Autodesk Inventor part; units mm, degrees
ref_plane "YZ Plane" through (0, 0, 0) normal (1, 0, 0) x (0, 1, 0)
ref_plane "XZ Plane" through (0, 0, 0) normal (0, 1, 0) x (-1, 0, 0)
ref_plane "XY Plane" through (0, 0, 0) normal (0, 0, 1) x (1, 0, 0)
sketch "Sketch1" plane through (0, 0, 0) normal (1, 0, 0) x (0, 1, 0)
  line L0 (0, 0) -> (15, 0)
  line L1 (15, 0) -> (12.3428, -7.0424)
  line L2 (12.3428, -7.0424) -> (2.9628, -13.5)
  line L3 (2.9628, -13.5) -> (-16.504, -16)
  line L4 (-16.504, -16) -> (-16.504, -11)
  line L5 (-16.504, -11) -> (-7.6685, -9.267)
  line L6 (-7.6685, -9.267) -> (-2.3251, -6.639)
  line L7 (-2.3251, -6.639) -> (0, 0)
  dimension "d0" = 15
  dimension "d24" = 16
  dimension "d27" = 5
extrude "Extrusion1" add sketch "Sketch1" along normal blind 20
sketch "Sketch2" plane through (0, 0, 0) normal (0, 0, 1) x (1, 0, 0)
  line L0 (-0.936, -0.2322) -> (7.6821, -18.3326)
  line L1 (7.6821, -18.3326) -> (-7.1135, -18.3326)
  line L2 (-7.1135, -18.3326) -> (-0.936, -0.2322)
extrude "Extrusion2" cut sketch "Sketch2" against normal blind 25
shell "Shell1" thickness 0.8 removed faces 2 at (6.6667, 5, 0) at (11.2076, -16.504, -14.3333)
sketch "Sketch3" plane through (0, 0, 0) normal (0, 0, 1) x (1, 0, 0)
  line L0 (0.8, 0.8476) -> (0.8, 14.1449)
  line L1 (0.8, 14.1449) -> (19.2, 14.1449)
  line L2 (19.2, 14.1449) -> (19.2, 0.8476)
  line L3 (19.2, 0.8476) -> (0.8, 0.8476)
  line L4 (0, 0) -> (0, 15)
  line L5 (0, 0) -> (20, 0)
  line L6 (20, 15) -> (20, 0)
  line L7 (0, 15) -> (20, 15)
  circle A0 centre (-3, 7.5) radius 1.25
  circle A1 centre (23, 7.5) radius 1.25
  line L8 (0, 0) -> (-6.2, 5.2024)
  line L9 (-6.2, 5.2024) -> (-6.2, 9.7976)
  line L10 (-6.2, 9.7976) -> (0, 15)
  line L11 (20, 15) -> (26.2, 9.7976)
  line L12 (26.2, 9.7976) -> (26.2, 5.2024)
  line L13 (26.2, 5.2024) -> (20, 0)
  line L14 (0, 0) -> (0, -1.5)
  line L15 (0, -1.5) -> (20, -1.5)
  line L16 (20, -1.5) -> (20, 0)
  dimension "d6" = 2.5
  dimension "d8" = 2.5
  dimension "d9" = 3
  dimension "d10" = 3
  dimension "d11" = 7.5
  dimension "d12" = 7.5
  dimension "d17" = 130
  dimension "d18" = 130
  dimension "d19" = 130
  dimension "d20" = 130
  dimension "d21" = 6.2
  dimension "d22" = 6.2
  dimension "d23" = 1.5
extrude "Extrusion3" add sketch "Sketch3" along normal blind 3
sketch "Sketch4" plane through (20, 0, 0) normal (1, 0, 0) x (0, 0, -1)
  line L0 (13.5, 2.9628) -> (7.0424, 12.3428)
  line L1 (7.0424, 12.3428) -> (0, 15)
  line L2 (0, 15) -> (9.6524, 15)
  line L3 (9.6524, 15) -> (11.8288, 5.3904)
extrude "Extrusion4" add sketch "Sketch4" against normal blind 20
sketch "Sketch5" plane through (0, 15, 3) normal (0, 1, 0) x (1, 0, 0)
  line L0 (0, 3) -> (0, 0)
  line L1 (20, 0) -> (0, 0)
  line L2 (20, 3) -> (20, 0)
  line L3 (20, 12.6524) -> (20, 3)
  line L4 (20, 12.6524) -> (0, 12.6524)
  line L5 (0, 3) -> (0, 12.6524)
extrude "Extrusion5" add sketch "Sketch5" along normal blind 1
properties part number "dysza_abs2"
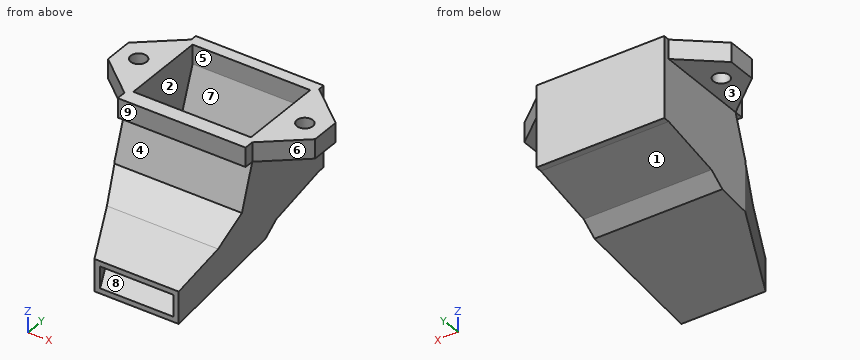
Source: CAD feature listing. Evaluate the final solid. Frame: model axes, mm. Face numbers are marked on the shaded views. A direction names the side the tool comes from. Give positions to 0.01 mm unless a question says otherwise; leave off trailing zeros. Order: outer loops, then holes, each group sorted by start corner. A loop starts at its lowest first (then second) coordinate and runs counter-clockwise, first axis right, second up. Notation, with made-up numbers: (-35.75, -5.75) -> (17.25, -5.75) arc R18 ccw to (17.25, 29.25) -> close; hole circle Ø3 at (-19.5, 74). An arc over 180 degrees is marked (long way). Use a Markdown table: item, result.
Q1. Material intervals for line 1 (X direction, y = 12, z = -3.75); line 2 (Y direction, x = 6, z = -0.5); line 3 (Y direction, x = -3, z = 0.7), sorted ascending. Write a range as [from, to].
A:
| item | result |
|---|---|
| line 1 | [0, 0.8], [19.2, 20] |
| line 2 | [-0.18, 0.67], [13.96, 16] |
| line 3 | [2.52, 6.25], [8.75, 12.48] |
Q2. First-contact query: P1, Ø2, axis at y = 10, z = -8.5, coming from the -X side; P2, Ø2, axis at y = 11.5, z = -12.5, coming from the -X side; P3, Ø0.8, axis at x = 6.5, y = 15.5, coming from the -Z side; P4, Ø3.5, axis at x = 10, z = 1, coming from the -Y side. Flat tips, straight axial feed; report the tip coordinate or a pass-through.
A:
| item | result |
|---|---|
| P1 | x = 0 |
| P2 | through |
| P3 | z = -9.65 |
| P4 | y = -1.5 |
Q3. Section C-C (y = 7.5). Return the cut outline in (x, z), and give its area (3 significant figures).
A:
| item | result |
|---|---|
| outline | (-6.2, 0) -> (-4.25, 0) -> (-4.25, 3) -> (-6.2, 3) -> close; (-1.75, 0) -> (0, 0) -> (0, -11.35) -> (20, -11.35) -> (20, 0) -> (21.75, 0) -> (21.75, 3) -> (19.2, 3) -> (19.2, -9.41) -> (0.8, -9.41) -> (0.8, 3) -> (-1.75, 3) -> close; (24.25, 0) -> (26.2, 0) -> (26.2, 3) -> (24.25, 3) -> close |
| area | 81.0 mm^2 |
Q4. Section B-B (z = -10.5). Return the cut outline in (x, y), and give its area (3 significant figures).
A:
| item | result |
|---|---|
| outline | (0, -2.2) -> (5.6, -13.95) -> (20, -13.95) -> (20, 11.26) -> (0, 11.26) -> close; hole (0.8, -2.02) -> (4.5, -9.8) -> (19.2, -9.8) -> (19.2, 5.91) -> (0.8, 5.91) -> close |
| area | 197 mm^2 |
Q5. Section D-D (y = 11). Return the cut outline in (x, z).
A:
| item | result |
|---|---|
| outline | (-4.77, 0) -> (0, 0) -> (0, -10.56) -> (20, -10.56) -> (20, 0) -> (24.77, 0) -> (24.77, 3) -> (19.2, 3) -> (19.2, -7) -> (0.8, -7) -> (0.8, 3) -> (-4.77, 3) -> close |
Q6. Access query for the marked faces 1, 2, 3, 4 and 5. Directions: +Z, -Z, +X, -X, +Y, -Y. A direction counts if a zero-diameter tool reaches every point of the face in a straight line with its end or side. Return the directions, or none.
A:
| item | result |
|---|---|
| face 1 | -Z, +X, -X, +Y |
| face 2 | none |
| face 3 | -Z, -X, +Y, -Y |
| face 4 | +X, -X, -Y |
| face 5 | +Z |
Q7. Pull-direction query (X, two-part tool) for the marked faces 6, 7, 8 and 9; classes: +X half, -X half, draft (parallel to the pull), parting line (faces both ways), or undercut.
A:
| item | result |
|---|---|
| face 6 | +X half |
| face 7 | undercut |
| face 8 | undercut |
| face 9 | draft |
